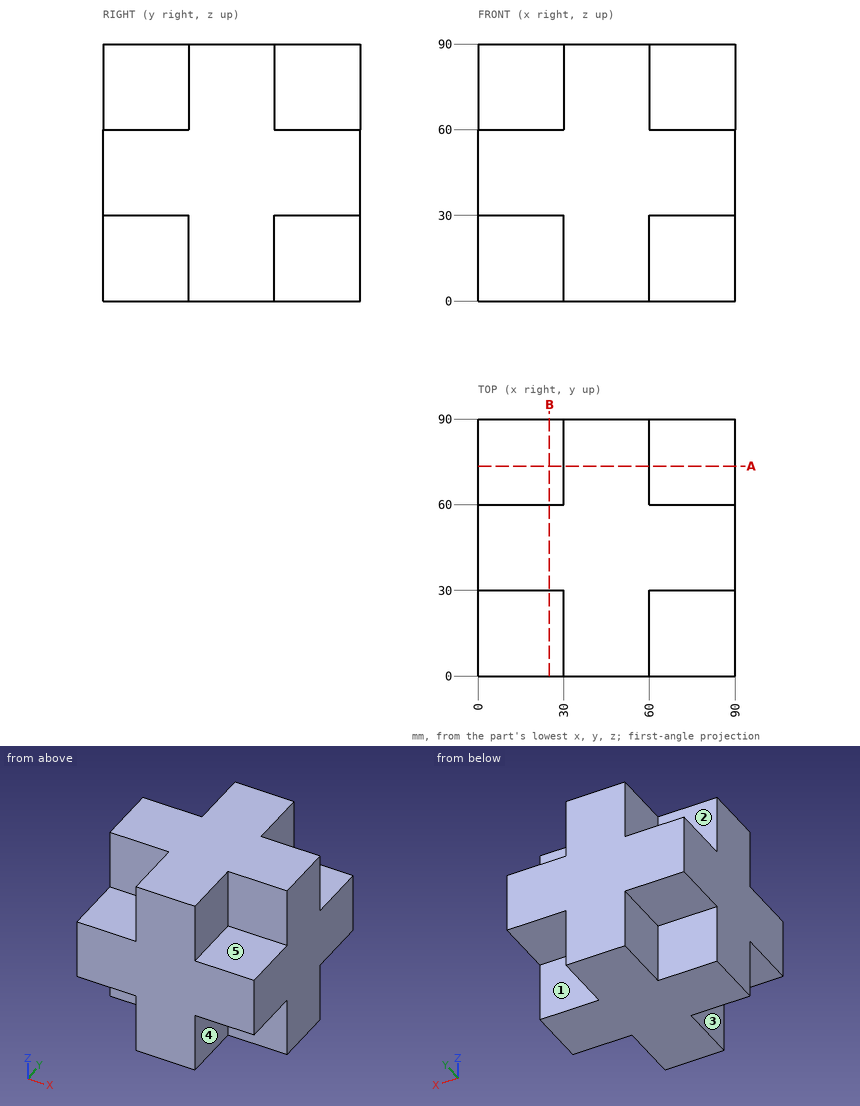
For this review, use the dimensioned drawing (mm, ordinates from the lowest corner) and the shaded views. A direction names the side the tool comes from. Coordinates: 2 decimals unless noted, no trailing zeros. Order: outer loops, then holes, each group sorted by start corner. A loop starts at its lowest first (then second) coordinate and runs counter-clockwise, first axis right, second up. Notation, with made-up numbers: (-24, -30) - (-18, -30) arc R5 ccw to (-18, -26) - close; hole circle Ø5 at (88, 16.25). An arc over 180 degrees is marked (long way). Answer as a JSON object with one key per item and string values. Group by question number.
1. We need section A-A on y = 73.5. State the section outline as (x, z) points.
2. For probe 1 along Y at (x, z) = (84.5, 78), list the stretches that pass through material, from the lowest coordinate up.
3. Clearance check with flat-ended pins moving along their axes: P1, Ø9, axis at x = 72.5, z = 16, coming from the +Y side; P2, Ø24, axis at x = 9.5, y = 14.5, coming from the -Z side; P3, Ø9, axis at x = 16.5, y = 18.5, coming from the +Z side. State where each tip first meets the part, or that it passes through.
4. For the marked faces 1, 2, 3, 4 and 5, list the 3-axis set-ups (+Z, -Z, +X, -X, +Y, -Y) from which the entire face can be reached by the end or side of a thin tool; tool diameter is ignored.
Final values:
{
 "1": {"outline": "(0, 30) - (30, 30) - (30, 0) - (60, 0) - (60, 30) - (90, 30) - (90, 60) - (60, 60) - (60, 90) - (30, 90) - (30, 60) - (0, 60) - close"},
 "2": {"probe 1": "30 to 60"},
 "3": {"P1": "y = 60", "P2": "z = 30", "P3": "z = 60"},
 "4": {"face 1": "-Z, +X, +Y", "face 2": "+Z, -X, +Y", "face 3": "-Z, -X, -Y", "face 4": "-Z, +X, -Y", "face 5": "+Z, +X, -Y"}
}
